```python
from build123d import *

# Parameters (mm, degrees)
BOSS_EXTRUDE1_DEPTH     = 5
SKETCH4_W               = 5
SKETCH4_H               = 6.1
CUT_EXTRUDE1_DEPTH      = 1
CHAMFER1_SIZE           = 3
CUT_EXTRUDE8_DEPTH      = 104.701494685
CUT_EXTRUDE8_DEPTH_BACK = 104.701494685
SKETCH13_R              = 0.25
CUT_EXTRUDE9_DEPTH      = 101.249688279
SKETCH14_W              = 0.27
SKETCH14_H              = 3
CUT_EXTRUDE11_DEPTH     = 101.204790305
SKETCH16_W              = 4.06
SKETCH16_H              = 3
CUT_EXTRUDE12_DEPTH     = 101.204790305
CHAMFER4_SIZE           = 1.25
CHAMFER7_SIZE           = 1.25
CHAMFER8_SIZE           = 1.25
CHAMFER9_SIZE           = 1.25


with BuildPart() as part:
    # Sketch1 → Boss-Extrude1 (new body)
    with BuildSketch(Plane.XY):
        with BuildLine():
            Line((0, -100), (-5, -100))
            Line((-5, -100), (-5, -60))
            Line((-5, -60), (-12, -5))
            Line((-12, -5), (-27, -5))
            Line((-27, -5), (-27, 0))
            Line((-27, 0), (-3, 0))
            Line((-3, 0), (-3, -37.2))
            ThreePointArc((-3, -37.2), (-2.179898987, -39.179898987), (-0.2, -40))
            Line((-0.2, -40), (0, -40))
            Line((0, -40), (0, -100))
        make_face()
    extrude(amount=BOSS_EXTRUDE1_DEPTH)

    # Sketch4 → Cut-Extrude1 (cut)
    with BuildSketch(Plane(origin=(0, 0, 0), x_dir=(0, 0, -1), z_dir=(1, 0, 0))):
        with Locations((-2.5, -92.95)):
            Rectangle(SKETCH4_W, SKETCH4_H)
        with Locations((-2.5, -82.85)):
            Rectangle(SKETCH4_W, SKETCH4_H)
        with Locations((-2.5, -72.75)):
            Rectangle(SKETCH4_W, SKETCH4_H)
        with Locations((-2.5, -62.65)):
            Rectangle(SKETCH4_W, SKETCH4_H)
        with Locations((-2.5, -52.55)):
            Rectangle(SKETCH4_W, SKETCH4_H)
        with Locations((-2.5, -42.45)):
            Rectangle(SKETCH4_W, SKETCH4_H)
    extrude(amount=-CUT_EXTRUDE1_DEPTH, mode=Mode.SUBTRACT)

    # Chamfer1
    chamfer1_edges = [part.edges().sort_by_distance(p)[0] for p in [
        (-5, -100, 2.5),
    ]]
    chamfer(chamfer1_edges, length=CHAMFER1_SIZE)

    # Sketch9 → Cut-Extrude8 (cut, two sides: drawn at the far end of the back side and taken through both)
    with BuildSketch(Plane.XY.offset(5).offset(-CUT_EXTRUDE8_DEPTH_BACK)):
        Polygon((157.782929128, -69.7), (-1, -69.7), (-5, -69.7), (-163.782929128, -69.7), (-163.782929128, 247.865858257), (157.782929128, 247.865858257), align=None)
    extrude(amount=CUT_EXTRUDE8_DEPTH + CUT_EXTRUDE8_DEPTH_BACK, mode=Mode.SUBTRACT)

    # Sketch13 → Cut-Extrude9 (cut, through all)
    with BuildSketch(Plane.XY.offset(5)):
        with Locations((-2.5, -71.2)):
            Circle(SKETCH13_R)
    extrude(amount=-CUT_EXTRUDE9_DEPTH, mode=Mode.SUBTRACT)

    # Sketch14 → Cut-Extrude11 (cut, through all)
    with BuildSketch(Plane(origin=(-1, 0, 0), x_dir=(0, 0, -1), z_dir=(1, 0, 0))):
        with Locations((-4.865, -71.2)):
            Rectangle(SKETCH14_W, SKETCH14_H)
        with Locations((-0.135, -71.2)):
            Rectangle(SKETCH14_W, SKETCH14_H)
    extrude(amount=-CUT_EXTRUDE11_DEPTH, mode=Mode.SUBTRACT)

    # Sketch16 → Cut-Extrude12 (cut, through all)
    with BuildSketch(Plane(origin=(-1, 0, 0), x_dir=(0, 0, -1), z_dir=(1, 0, 0))):
        with Locations((-2.5, -71.2)):
            Rectangle(SKETCH16_W, SKETCH16_H)
    extrude(amount=-CUT_EXTRUDE12_DEPTH, mode=Mode.SUBTRACT)

    # Chamfer4
    chamfer4_edges = [part.edges().sort_by_distance(p)[0] for p in [
        (-1, -69.7, 4.63),
    ]]
    chamfer(chamfer4_edges, length=CHAMFER4_SIZE)

    # Chamfer7
    chamfer7_edges = [part.edges().sort_by_distance(p)[0] for p in [
        (-1, -69.7, 0.37),
    ]]
    chamfer(chamfer7_edges, length=CHAMFER7_SIZE)

    # Chamfer8
    chamfer8_edges = [part.edges().sort_by_distance(p)[0] for p in [
        (-5, -69.7, 4.63),
    ]]
    chamfer(chamfer8_edges, length=CHAMFER8_SIZE)

    # Chamfer9
    chamfer9_edges = [part.edges().sort_by_distance(p)[0] for p in [
        (-5, -69.7, 0.37),
    ]]
    chamfer(chamfer9_edges, length=CHAMFER9_SIZE)


solid = part.part
```
Can you work these out from the model? Positions are in its coordinate system, mm. A direction names the side the tool comes from. Coordinates: 2 decimals unless noted, no trailing zeros. Write each loop counter-clockwise with the first axis right and the second up, starting at its lowest first coordinate (ties: lowest second). Pieces come first, ordered by that corner, then holes. Notation, with made-up numbers: (57.25, 69) - (82.25, 69) arc R5 cw to (82.25, 77) - close; hole circle Ø4 at (-15.75, 15). An arc over 180 degrees is marked (long way). Return JSON: item names as keys, results as strings.
Q1. If we section it at A-A (y = -71.2): Please give me the cut outline in (x, z), then the cut area to 3 significant figures.
Computed values:
{"outline": "(-5, 0.27) - (-2.75, 0.27) - (-2.75, 0.47) - (-5, 0.47) - close; (-5, 4.53) - (-2.75, 4.53) - (-2.75, 4.73) - (-5, 4.73) - close; (-2.25, 0.27) - (-1, 0.27) - (-1, 0.47) - (-2.25, 0.47) - close; (-2.25, 4.53) - (-1, 4.53) - (-1, 4.73) - (-2.25, 4.73) - close", "area": "1.40 mm2"}
Q2. On a 3-axis mill with a long thin cutter (end or side, diameter ignored), from which of +Z, -Z, +X, -X, +Y, -Y can I reach the whole of each face in a straight line? I mean faces 4 (the flat face through (-3, -71, 4.53)), 5 (the flat face through (-0.5, -75.8, 2.5)), 6 (the flat face through (-3, -71, 0.27)). Say none if no direction works.
Computed values:
{"face 4": "+X, -X, +Y", "face 5": "+Z, -Z, +X, +Y", "face 6": "-Z, +X, -X, +Y"}
Q3. Please list where these lines run through material, in increasing order: L1, parallel to Y at x = -0.6, z = 2.2; L2, parallel to X at y = -71.2, z = 4.6; L3, parallel to Z at x = -3.3, y = -72. Write a range as from..to.
Computed values:
{"L1": "y = -100..-96, -89.9..-85.9, -79.8..-75.8", "L2": "x = -5..-2.75, -2.25..-1", "L3": "z = 0.27..0.47, 4.53..4.73"}
Q4. If we section it at C-C (z = 1.6): Please give me the cut outline in (x, y), then the cut area to 3 significant figures.
Computed values:
{"outline": "(-5, -97) - (-2, -100) - (0, -100) - (0, -96) - (-1, -96) - (-1, -89.9) - (0, -89.9) - (0, -85.9) - (-1, -85.9) - (-1, -79.8) - (0, -79.8) - (0, -75.8) - (-1, -75.8) - (-1, -72.7) - (-5, -72.7) - close", "area": "117 mm2"}
Q5. Thinking about a two-plate mould opening in Y: for faces 1 (the flat face through (-0.5, -89.9, 2.5)), 2 (the flat face through (-4, -98, 2)), 3 (the flat face through (-5, -84, 2)), which applies, +Y half, -Y half, draft (parallel to the pull), parting line (faces both ways), or undercut?
Computed values:
{"face 1": "undercut", "face 2": "-Y half", "face 3": "draft"}
Q6. I'm going to push flat-ended pins straight in: pin 1 Ø1.1 at (x, z) = (-0.5, 2.5) entering from +Y; pin 2 Ø1 at (x, y) = (-1.5, -93) entering from -Z; pin 3 Ø0.8 at (x, z) = (-0.5, 3.5) entering from +Y; pin 4 Ø2.5 at (y, z) = (-82, 3.5) entering from +X. Where does each tip first touch, or does it pass through?
Computed values:
{"pin 1": "stops at y = -72.7", "pin 2": "stops at z = 0", "pin 3": "stops at y = -75.8", "pin 4": "stops at x = -1"}
Q7. If we section it at B-B (x = -2.5): Please give me the cut outline in (y, z), then the cut area to 3 significant figures.
Computed values:
{"outline": "(-99.5, 0) - (-72.7, 0) - (-72.7, 0.27) - (-71.45, 0.27) - (-71.45, 0.47) - (-72.7, 0.47) - (-72.7, 4.53) - (-71.45, 4.53) - (-71.45, 4.73) - (-72.7, 4.73) - (-72.7, 5) - (-99.5, 5) - close; (-70.95, 0.27) - (-69.7, 0.27) - (-69.7, 0.47) - (-70.95, 0.47) - close; (-70.95, 4.53) - (-69.7, 4.53) - (-69.7, 4.73) - (-70.95, 4.73) - close", "area": "135 mm2"}
